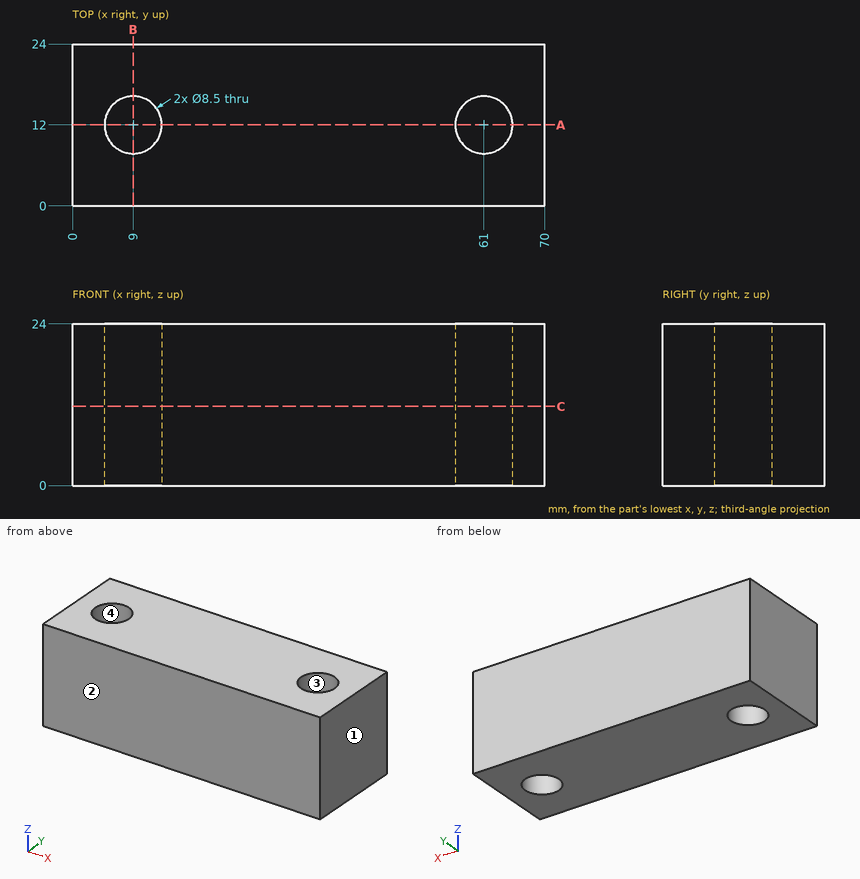
Job drawing, mm, ordinate dimensions from the low corner. One solid piece. Round coordinates to 2 decimals unless told otherwise and drop trailing zeros. Write each loop counter-clockwise with the first axis right and the second up, starting at its lowest first coordinate (ties: lowest second). Pieces come first, ordered by that corner, then holes. Notation, with made-up numbers: M 56.5,35.25 L 74.5,35.25 A36 cw 74.5,74.25 Z; hole C 3,4 d9. An arc over 180 degrees is marked long. Return JSON: item names as keys, results as strings. Group by question number.
(1) Saw through at C-C on z = 11.75. Write the cut outline in (x, y), then the cut area to 3 significant figures.
(2) Saw through at B-B on x = 9. Write the cut outline in (y, z), then the cut area to 3 significant figures.
(3) Drill centre lines: probe 1 along Y at (x, z) = (61, 18.25); probe 2 along X at (y, z) = (14.5, 15.5); probe 3 along Y at (x, z) = (59, 12.5). Where is each one in solid material? Low to high.
(4) Saw through at A-A on y = 12. Write the cut outline in (x, z).
(5) Two-plate mould, pull along X, no slides. Class the marked faces 1, 2, 3 and 4: +X half, -X half, draft (parallel to the pull), parting line (faces both ways), or undercut.
Returned:
{
 "1": {"outline": "M 0,0 L 70,0 L 70,24 L 0,24 Z; hole C 9,12 d8.5; hole C 61,12 d8.5", "area": "1,570 mm²"},
 "2": {"outline": "M 0,0 L 7.75,0 L 7.75,24 L 0,24 Z; M 16.25,0 L 24,0 L 24,24 L 16.25,24 Z", "area": "372 mm²"},
 "3": {"probe 1": "0 to 7.75, 16.25 to 24", "probe 2": "0 to 5.56, 12.44 to 57.56, 64.44 to 70", "probe 3": "0 to 8.25, 15.75 to 24"},
 "4": {"outline": "M 0,0 L 4.75,0 L 4.75,24 L 0,24 Z; M 13.25,0 L 56.75,0 L 56.75,24 L 13.25,24 Z; M 65.25,0 L 70,0 L 70,24 L 65.25,24 Z"},
 "5": {"face 1": "+X half", "face 2": "draft", "face 3": "undercut", "face 4": "undercut"}
}
